from build123d import *

# Parameters (mm, degrees)
F1_DEPTH = 25.4
F1_TAPER = -3
F2_R     = 43.1135543891
F3_DEPTH = 25.4
F3_TAPER = -3
F4_R     = 16.6756638842
F5_DEPTH = 25.4
F5_TAPER = -3


with BuildPart() as f1:
    # F0 (on Front) → F1 (new body)
    with BuildSketch(Plane.XZ):
        Polygon((129.7552857443, 7.7033717296), (-71.5489584847, 108.5196878651), (-58.2063272595, -116.2230595946), align=None)
    extrude(amount=F1_DEPTH, taper=F1_TAPER)

    # F2 (on face) → F3 (join)
    with BuildSketch(Plane(origin=(0, 0, 0), x_dir=(-1, 0, 0), z_dir=(0, 1, 0))):
        Circle(F2_R)
    extrude(amount=F3_DEPTH, taper=F3_TAPER)

    # F4 (on face) → F5 (join)
    with BuildSketch(Plane(origin=(0, 0, 0), x_dir=(-1, 0, 0), z_dir=(0, 1, 0))):
        Circle(F4_R)
    extrude(amount=F5_DEPTH, taper=F5_TAPER)


solid = f1.part
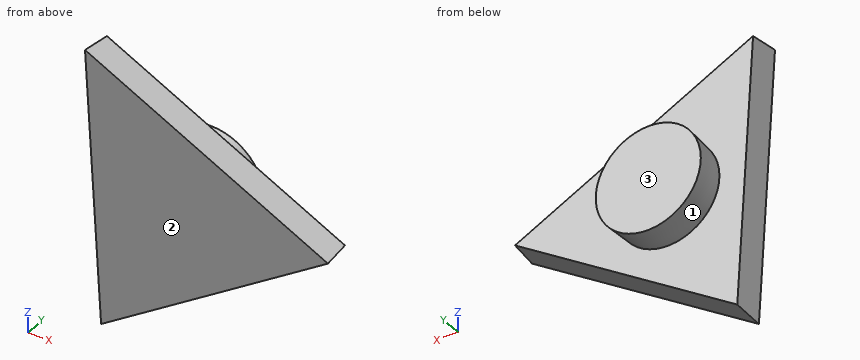
The listing builds one solid part. Answer for the finished solid, in the listing's coordinates (mm). Face numbers are marked on the shaded views. Coordinates: 2 decimals unless noted, no trailing zeros. Write each loop counter-clockwise with the first axis right and the second up, starting at its lowest first coordinate (ties: lowest second). Pieces come first, ordered by that corner, then holes. Notation, with made-up numbers: (16, 1) -> (38, 1) arc R23 ccw to (38, 29) -> close; hole circle Ø10 at (36.5, 4.25). An arc over 180 degrees is marked (long way). One line per question, with ' | ' between items.
1. Section B-B (y = 5) is taken. Determine the outline of the cut face in (x, z).
Verdict:
outline: circle Ø86.75 at (0, 0)
2. Section A-A (y = 21.5) is taken. Determine the outline of the cut face in (x, z), and give its area (3 significant figures).
Verdict:
outline: circle Ø88.48 at (0, 0) | area: 6,150 mm^2
3. Straight lines are drawn through the part: line 1 (Y direction, x = 34, z = -53); line 2 (Z direction, x = -52.5, y = -2); line 3 (X direction, y = -7, z = 30). For each, find the intervals that lie inside material, in ascending order.
Verdict:
line 1: y = -25.4 to 0 | line 2: z = -112.59 to 99.1 | line 3: x = -67.25 to 86.05
4. For a pull along Y with two mould halves and no side action, classify the marked faces 1, 2 and 3 as released by +Y, released by -Y, zero draft, split by the parting line, or undercut.
Verdict:
face 1: undercut | face 2: released by -Y | face 3: released by +Y
5. Given pin 1 Ø10 at (x, z) = (-1, -55) entering from +Y; pin 2 Ø12 at (y, z) = (2, -69.5) entering from -X; pin 3 Ø3 at (y, z) = (-19.5, -5) entering from +X, each flat-ended and moving along its own axis, determine where each tip first touches the part or whether it passes through.
Verdict:
pin 1: stops at y = 0 | pin 2: stops at x = -61.35 | pin 3: stops at x = 114.62
